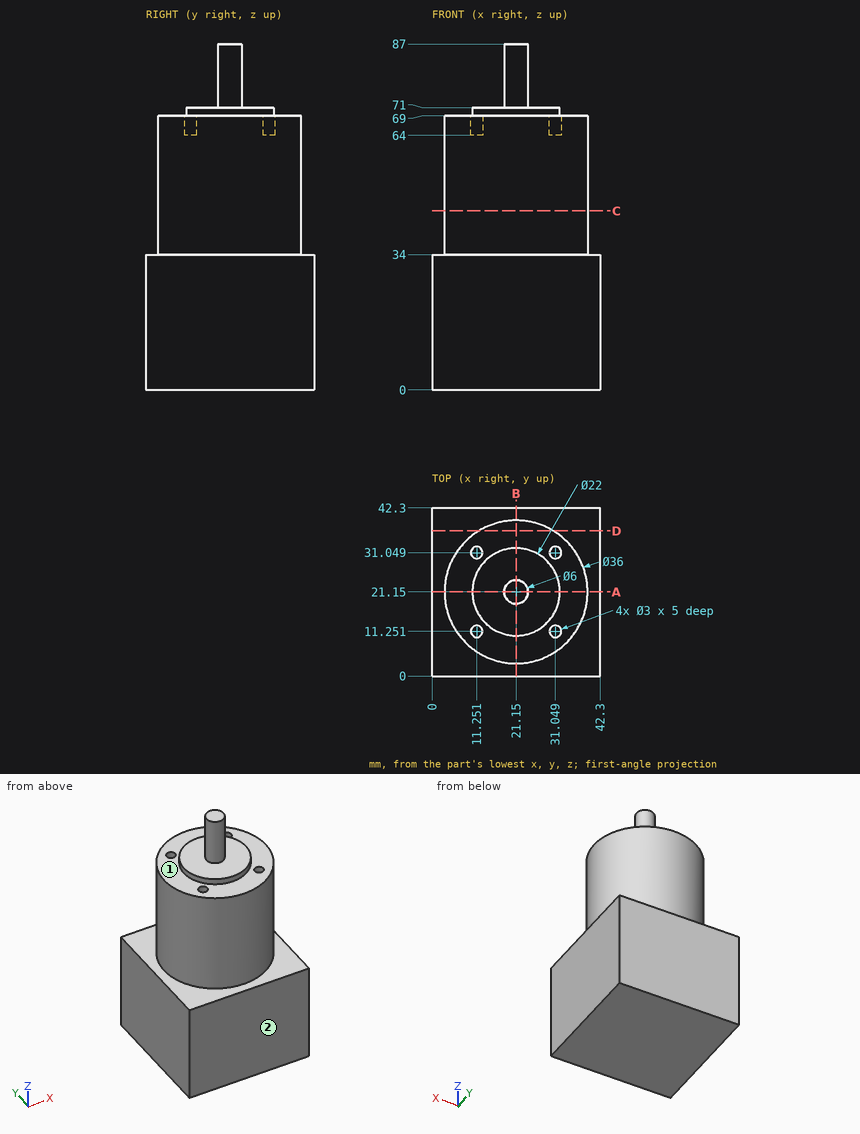
Job drawing, mm, ordinate dimensions from the low corner. One solid piece. A direction names the side the tool comes from. Coordinates: 2 decimals unless noted, no trailing zeros. Write each loop counter-clockwise with the first axis right and the second up, starting at its lowest first coordinate (ties: lowest second). Pieces come first, ordered by that corner, then holes. Notation, with made-up numbers: (8.25, 30.5) -> (14.25, 30.5) arc R22 cw to (14.25, 50.5) -> close; hole circle Ø10 at (-30, 4.25). An arc over 180 degrees is marked (long way). Use CSV: the item, a comma, the result in double quotes. Start each with the question number.
Item 1: Band-saw the part on C-C, the plane z = 45. Write the cut outline in (x, y).
Item 2: Drop flat-ended pins along their axis: P1, Ø0.9, axis at x = 11, y = 31, coming from the +Z side; P2, Ø8, axis at x = 14, y = 26, coming from the -Z side; P3, Ø2, axis at x = 4.5, y = 34.5, coming from the +Z side; P4, Ø1.5, axis at x = 11, y = 12, coming from the +Z side. Give the stop position or say it passes through.
Item 3: Tool access for the marked faces 1 and 2: list every direction of +Z, -Z, +X, -X, +Y, -Y with a clear straight run to the whole face (end or side of a thin tool).
Item 4: Band-saw the part on D-D, the plane y = 36.5. Write the cut outline in (x, z), plus the area to 3 significant figures.
Item 5: Wall check: probe 1 along Z at (x, y) = (37.5, 4.5); probe 2 along Z at (x, y) = (17, 19); probe 3 along X at (y, z) = (30.5, 45.5). Give the ranges that are in metal, low to high.
Item 6: Band-saw the part on A-A, the plane y = 21.15. Write the cut outline in (x, z).
Response values:
1,outline,"circle Ø36 at (21.15, 21.15)"
2,P1,"stops at z = 64"
2,P2,"stops at z = 0"
2,P3,"stops at z = 34"
2,P4,"stops at z = 69"
3,face 1,"+Z"
3,face 2,"+Z, -Z, +X, -X, -Y"
4,outline,"(0, 0) -> (42.3, 0) -> (42.3, 34) -> (30.55, 34) -> (30.55, 69) -> (11.75, 69) -> (11.75, 34) -> (0, 34) -> close"
4,area,"2,100 mm2"
5,probe 1,"z = 0 to 34"
5,probe 2,"z = 0 to 71"
5,probe 3,"x = 5.77 to 36.53"
6,outline,"(0, 0) -> (42.3, 0) -> (42.3, 34) -> (39.15, 34) -> (39.15, 69) -> (32.15, 69) -> (32.15, 71) -> (24.15, 71) -> (24.15, 87) -> (18.15, 87) -> (18.15, 71) -> (10.15, 71) -> (10.15, 69) -> (3.15, 69) -> (3.15, 34) -> (0, 34) -> close"
